For this review, take the finished solid that the model builds, in its own axes (mm). A direction names the side the tool comes from. Round coordinates to 2 decimals unless told otherwise and drop trailing zeros. Write each loop counter-clockwise with the first axis right and the second up, starting at its lowest first coordinate (ties: lowest second). Pieces come first, ordered by that corner, then holes. Notation, with made-up numbers: (25.25, -19.5) - (46.25, -19.5) arc R16 ccw to (46.25, 3.5) - close; hole circle Ø2 at (69, -8.75). An arc over 180 degrees is marked (long way). One line per item, written item: value. Start each with the question number.
Q1. For probe 1 along Y at (x, z) = (0.25, 6) (3 decimals); probe 2 along X at (y, z) = (-2.5, 0.5); probe 3 along Y at (x, z) = (-5.5, 5.25), list the stretches that pass through material, from the lowest coordinate up.
Q2. Tool access review of faces 1 (the face through (-6.07, 4.32, 4.93)), 2 (the face through (4.5, 5, 5)): name each direction out of +Z, -Z, +X, -X, +Y, -Y from which nothing blocks a thin tool from reaching the whole face with its end or side.
Q3. Add section B-B on y = 8.75. Write out the cut boundary in (x, z), and give its area (3 significant figures).
Q4. Add section C-C on y = -1.25. Write out the cut boundary in (x, z).
Q5. Clearance check with flat-ended pins moving along their axes: pin 1 Ø5 at (x, z) = (-8.5, 4) entering from +Y; pin 2 Ø1.5 at (x, z) = (4.5, 6) entering from +Y; pin 3 Ø4 at (y, z) = (-6, 2) entering from -X. State where each tip first meets the part, or that it passes through.
Q6. Mouldability with a two-part tool opening along X and no side actions: class faces 3 (the face through (-1.72, -6.98, 4.93)), 4 (the face through (-5.7, 5, 5)), 5 (the face through (-2, -5, 0)) as +X half, -X half, draft (parallel to the pull), parting line (faces both ways), or undercut.
Q7. Add section A-A on x = 0. Write out the cut boundary in (y, z).
```python
from build123d import *

# Parameters (mm, degrees)
F1_DEPTH = 10
F2_T     = -1.2


with BuildPart() as f1:
    # F0 (on Top) → F1 (new body)
    with BuildSketch(Plane.XY):
        with BuildLine():
            ThreePointArc((-5.066449, 0.370803), (-4.939368, 1.187032), (-4.681679, 1.971873))
            ThreePointArc((-4.681679, 1.971873), (-4.674597, 2.264385), (-4.868556, 2.483458))
            Line((-4.868556, 2.483458), (-5.198977, 2.652007))
            ThreePointArc((-5.198977, 2.652007), (-5.401697, 2.897981), (-5.360275, 3.214024))
            ThreePointArc((-5.360275, 3.214024), (-4.962027, 3.800103), (-4.5, 4.337338))
            Line((-4.5, 4.337338), (-4.5, 6))
            ThreePointArc((-4.5, 6), (-5.964466, 9.535534), (-9.5, 11))
            ThreePointArc((-9.5, 11), (-10.56066, 10.56066), (-11, 9.5))
            Line((-11, 9.5), (-11, 0))
            ThreePointArc((-11, 0), (0, -11), (11, 0))
            Line((11, 0), (11, 9.5))
            ThreePointArc((11, 9.5), (10.56066, 10.56066), (9.5, 11))
            ThreePointArc((9.5, 11), (5.964466, 9.535534), (4.5, 6))
            Line((4.5, 6), (4.5, 4.337338))
            ThreePointArc((4.5, 4.337338), (4.941382, 3.82691), (5.325163, 3.271872))
            ThreePointArc((5.325163, 3.271872), (5.370003, 2.956296), (5.169959, 2.708141))
            Line((5.169959, 2.708141), (4.841382, 2.536025))
            ThreePointArc((4.841382, 2.536025), (4.649807, 2.314864), (4.660055, 2.022447))
            ThreePointArc((4.660055, 2.022447), (4.932869, 1.213755), (5.066449, 0.370803))
            ThreePointArc((5.066449, 0.370803), (5.193058, 0.107016), (5.465382, 0))
            Line((5.465382, 0), (5.836309, 0))
            ThreePointArc((5.836309, 0), (6.128661, -0.126998), (6.235373, -0.42735))
            ThreePointArc((6.235373, -0.42735), (6.155048, -1.085301), (6.005496, -1.731045))
            ThreePointArc((6.005496, -1.731045), (5.802494, -1.976786), (5.484336, -1.996135))
            Line((5.484336, -1.996135), (5.135779, -1.869271))
            ThreePointArc((5.135779, -1.869271), (4.843276, -1.876693), (4.634083, -2.081268))
            ThreePointArc((4.634083, -2.081268), (4.399409, -2.54), (4.119473, -2.972599))
            ThreePointArc((4.119473, -2.972599), (4.046902, -3.256054), (4.186725, -3.51308))
            Line((4.186725, -3.51308), (4.470872, -3.751507))
            ThreePointArc((4.470872, -3.751507), (4.613194, -4.036714), (4.501877, -4.33539))
            ThreePointArc((4.501877, -4.33539), (4.017423, -4.787778), (3.487783, -5.186316))
            ThreePointArc((3.487783, -5.186316), (3.174314, -5.244077), (2.918154, -5.054392))
            Line((2.918154, -5.054392), (2.732691, -4.73316))
            ThreePointArc((2.732691, -4.73316), (2.50385, -4.550828), (2.2121, -4.573075))
            ThreePointArc((2.2121, -4.573075), (1.737462, -4.773639), (1.244949, -4.925089))
            ThreePointArc((1.244949, -4.925089), (1.007156, -5.09558), (0.949054, -5.382351))
            Line((0.949054, -5.382351), (1.013464, -5.747642))
            ThreePointArc((1.013464, -5.747642), (0.939162, -6.057606), (0.661903, -6.214852))
            ThreePointArc((0.661903, -6.214852), (0, -6.25), (-0.661903, -6.214852))
            ThreePointArc((-0.661903, -6.214852), (-0.939162, -6.057606), (-1.013464, -5.747642))
            Line((-1.013464, -5.747642), (-0.949054, -5.382351))
            ThreePointArc((-0.949054, -5.382351), (-1.007156, -5.09558), (-1.244949, -4.925089))
            ThreePointArc((-1.244949, -4.925089), (-1.737462, -4.773639), (-2.2121, -4.573075))
            ThreePointArc((-2.2121, -4.573075), (-2.50385, -4.550828), (-2.732691, -4.73316))
            Line((-2.732691, -4.73316), (-2.918154, -5.054392))
            ThreePointArc((-2.918154, -5.054392), (-3.174314, -5.244077), (-3.487783, -5.186316))
            ThreePointArc((-3.487783, -5.186316), (-4.017423, -4.787778), (-4.501877, -4.33539))
            ThreePointArc((-4.501877, -4.33539), (-4.613194, -4.036714), (-4.470872, -3.751507))
            Line((-4.470872, -3.751507), (-4.186725, -3.51308))
            ThreePointArc((-4.186725, -3.51308), (-4.046902, -3.256054), (-4.119473, -2.972599))
            ThreePointArc((-4.119473, -2.972599), (-4.399409, -2.54), (-4.634083, -2.081268))
            ThreePointArc((-4.634083, -2.081268), (-4.843276, -1.876693), (-5.135779, -1.869271))
            Line((-5.135779, -1.869271), (-5.484336, -1.996135))
            ThreePointArc((-5.484336, -1.996135), (-5.802494, -1.976786), (-6.005496, -1.731045))
            ThreePointArc((-6.005496, -1.731045), (-6.155048, -1.085301), (-6.235373, -0.42735))
            ThreePointArc((-6.235373, -0.42735), (-6.128661, -0.126998), (-5.836309, 0))
            Line((-5.836309, 0), (-5.465382, 0))
            ThreePointArc((-5.465382, 0), (-5.193058, 0.107016), (-5.066449, 0.370803))
        make_face()
    extrude(amount=F1_DEPTH)

    # F2
    f2_openings = [f1.faces().sort_by_distance(p)[0] for p in [
        (-1.187768, -6.244675, 10),
        (-1.187768, -6.244675, 0),
    ]]
    offset(amount=F2_T, openings=f2_openings)


solid = f1.part
```
Result set:
1. probe 1: y = -10.997 to -9.797, -7.446 to -6.245
1. probe 2: x = -10.71 to -9.48, -6.96 to -4.42, 4.42 to 6.96, 9.48 to 10.71
1. probe 3: y = -9.53 to -8.11, -5.01 to -2, 0 to 9
2. face 1: +Z, -Z
2. face 2: +Z, -Z, +Y
3. outline: (-11, 0) - (-9.8, 0) - (-9.8, 10) - (-11, 10) - close; (-6.88, 0) - (-5.32, 0) - (-5.32, 10) - (-6.88, 10) - close; (5.32, 0) - (6.88, 0) - (6.88, 10) - (5.32, 10) - close; (9.8, 0) - (11, 0) - (11, 10) - (9.8, 10) - close
3. area: 55.1 mm^2
4. outline: (-10.93, 0) - (-9.72, 0) - (-9.72, 10) - (-10.93, 10) - close; (-7.34, 0) - (-6.12, 0) - (-6.12, 10) - (-7.34, 10) - close; (6.12, 0) - (7.34, 0) - (7.34, 10) - (6.12, 10) - close; (9.72, 0) - (10.93, 0) - (10.93, 10) - (9.72, 10) - close
5. pin 1: stops at y = 11
5. pin 2: stops at y = 8.63
5. pin 3: stops at x = -10.25
6. face 3: undercut
6. face 4: undercut
6. face 5: draft
7. outline: (-11, 0) - (-9.8, 0) - (-9.8, 10) - (-11, 10) - close; (-7.45, 0) - (-6.25, 0) - (-6.25, 10) - (-7.45, 10) - close
